Part model, mm, in its own coordinate system. A direction names the side the tool comes from. Coordinates: 2 decimals unless noted, no trailing zeros. Write each loop counter-clockwise with the first axis right and the second up, starting at its lowest first coordinate (ties: lowest second). Pieces come first, ordered by that corner, then holes. Notation, with made-up numbers: (-13.5, 80.25) - (8.5, 80.25) arc R24 ccw to (8.5, 111.25) - close; hole circle Ø2 at (86.25, 59.25). An arc over 180 degrees is marked (long way). Use a Markdown table: item, result.
```python
from build123d import *

# Parameters (mm, degrees)
SKETCH5_W            = 30
SKETCH5_H            = 80
BOSS_EXTRUDE4_DEPTH  = 20
SKETCH6_W            = 8
SKETCH6_H            = 5
BOSS_EXTRUDE5_DEPTH  = 5
SKETCH9_W            = 15
SKETCH9_H            = 22
BOSS_EXTRUDE10_DEPTH = 70
SKETCH14_W           = 15
SKETCH14_H           = 24
CUT_EXTRUDE1_DEPTH   = 18
FILLET1_R            = 2
FILLET2_R            = 10
FILLET4_R            = 2
FILLET6_R            = 2
SKETCH18_W           = 10
SKETCH18_H           = 18
BOSS_EXTRUDE11_DEPTH = 80
BOSS_EXTRUDE12_DEPTH = 10
CUT_EXTRUDE4_DEPTH   = 22


with BuildPart() as part:
    # Sketch5 → Boss-Extrude4 (new body)
    with BuildSketch(Plane(origin=(0, 0, 0), x_dir=(1, 0, 0), z_dir=(0, 1, 0))):
        Rectangle(SKETCH5_W, SKETCH5_H)
    extrude(amount=BOSS_EXTRUDE4_DEPTH)

    # Sketch6 → Boss-Extrude5 (add)
    with BuildSketch(Plane(origin=(0, 20, 0), x_dir=(1, 0, 0), z_dir=(0, 1, 0))):
        with Locations((8, 35.5)):
            Rectangle(SKETCH6_W, SKETCH6_H)
    extrude(amount=BOSS_EXTRUDE5_DEPTH)

    # Sketch9 → Boss-Extrude10 (add)
    with BuildSketch(Plane(origin=(0, 0, 0), x_dir=(1, 0, 0), z_dir=(0, 1, 0))):
        with Locations((-22.5, -24)):
            Rectangle(SKETCH9_W, SKETCH9_H)
    extrude(amount=BOSS_EXTRUDE10_DEPTH)

    # Sketch14 → Cut-Extrude1 (cut)
    with BuildSketch(Plane(origin=(0, 0, 13), x_dir=(-1, 0, 0), z_dir=(0, 0, -1))):
        with Locations((22.5, 54)):
            Rectangle(SKETCH14_W, SKETCH14_H)
    extrude(amount=-CUT_EXTRUDE1_DEPTH, mode=Mode.SUBTRACT)

    # Fillet1
    fillet1_edges = [part.edges().sort_by_distance(p)[0] for p in [
        (-15, 10, -40),
        (15, 10, -40),
        (15, 10, 40),
        (-15, 10, 40),
    ]]
    fillet(fillet1_edges, radius=FILLET1_R)

    # Fillet2
    fillet2_edges = [part.edges().sort_by_distance(p)[0] for p in [
        (-15, 10, 13),
    ]]
    fillet(fillet2_edges, radius=FILLET2_R)

    # Fillet4
    fillet4_edges = [part.edges().sort_by_distance(p)[0] for p in [
        (-30, 68, 13),
    ]]
    fillet(fillet4_edges, radius=FILLET4_R)

    # Fillet6
    fillet6_edges = [part.edges().sort_by_distance(p)[0] for p in [
        (-22.5, 70, 35),
        (-30, 70, 25),
        (-15, 70, 24),
        (-21.5, 70, 13),
        (-29.414213562, 70, 13.585786438),
    ]]
    fillet(fillet6_edges, radius=FILLET6_R)

    # Sketch18 → Boss-Extrude11 (add)
    with BuildSketch(Plane(origin=(0, 0, 0), x_dir=(-1, 0, 0), z_dir=(0, -1, 0))):
        with Locations((20, 13)):
            Rectangle(SKETCH18_W, SKETCH18_H)
    extrude(amount=-BOSS_EXTRUDE11_DEPTH)

    # Sketch19 → Boss-Extrude12 (add)
    with BuildSketch(Plane(origin=(0, 80, 0), x_dir=(1, 0, 0), z_dir=(0, 1, 0))):
        Polygon((-15, 22), (5, 22), (5, 14.741263634), (5, 6.741263634), (5, 4), (-15, 4), (-15, 6.741263634), (-15, 14.741263634), align=None)
    extrude(amount=-BOSS_EXTRUDE12_DEPTH)

    # Sketch20 → Cut-Extrude4 (cut)
    with BuildSketch(Plane(origin=(5, 0, 0), x_dir=(0, 0, -1), z_dir=(1, 0, 0))):
        Polygon((20, 80), (6, 80), (6, 78), (4, 78), (4, 72), (6, 72), (6, 70), (20, 70), (20, 72), (22, 72), (22, 78), (20, 78), align=None)
    extrude(amount=-CUT_EXTRUDE4_DEPTH, mode=Mode.SUBTRACT)


solid = part.part
```
Item 1: Two-plate mould, pull along Z, no slides. Class faces 5 (the face through (0, 10, 40)), 6 (the face through (-15, 10, 0)), 7 (the face through (4, 22, -35)): pulls with the +Z half, pulls with the -Z half, needs draft (parallel to the pull), parting line crosses it, or undercut.
From the geometry:
| item | result |
|---|---|
| face 5 | pulls with the +Z half |
| face 6 | undercut |
| face 7 | needs draft |
Item 2: Band-saw the part on D-D, the plane x = -21.5. Give the cut face in (y, z).
From the geometry:
| item | result |
|---|---|
| outline | (0, -22) - (80, -22) - (80, -4) - (0, -4) - close; (0, 12.37) - (20, 12.37) - (20, 13) - (42, 13) - (42, 31) - (66, 31) - (66, 13) - (68, 13) arc R2 ccw to (70, 15) - (70, 33) arc R2 ccw to (68, 35) - (0, 35) - close |
Item 3: Drop flat-ended pins along their axis: P1, Ø4, axis at x = 8, y = 21.5, coming from the -Z side; P2, Ø20, axis at y = 37.5, z = -9.5, coming from the +X side; P3, Ø1, axis at x = -16, z = -10, coming from the +Y side; P4, Ø12, axis at x = -22.5, y = 56, coming from the -Z side. Give the stop position or say it passes through.
From the geometry:
| item | result |
|---|---|
| P1 | z = -40 |
| P2 | x = -15 |
| P3 | y = 70 |
| P4 | z = -22 |
Item 4: Band-saw the part on C-C, the plane y = 65. Give the cut face in (x, z).
From the geometry:
| item | result |
|---|---|
| outline | (-30, 31) - (-15, 31) - (-15, 35) - (-30, 35) - close; (-25, -22) - (-15, -22) - (-15, -4) - (-25, -4) - close |
Item 5: Which spindle directions (+Z, -Z, +X, -X, +Y, -Y) get a long thin tool onto all of the face, cutting with end or side? Do faces 1 (the face through (-22, 67, 13)), 2 (the face through (-18.01, 10.14, 10.15)), 3 (the face through (-22, 66, 22)), 4 (the face through (-15, 33, 27)). Say none if no direction does.
From the geometry:
| item | result |
|---|---|
| face 1 | +X, -X, +Y |
| face 2 | -X, +Y, -Y |
| face 3 | +X, -X |
| face 4 | +Z, -Z, +X, +Y |
Item 6: Band-saw the part on B-B, the plane x = -1. Give the cut face in (y, z), then the cut area to 3 significant figures.
From the geometry:
| item | result |
|---|---|
| outline | (0, -40) - (20, -40) - (20, 40) - (0, 40) - close; (70, -22) - (72, -22) - (72, -20) - (70, -20) - close; (70, -6) - (72, -6) - (72, -4) - (70, -4) - close; (78, -22) - (80, -22) - (80, -20) - (78, -20) - close; (78, -6) - (80, -6) - (80, -4) - (78, -4) - close |
| area | 1,620 mm^2 |
Item 7: Drill centre lines: probe 1 along Z at (x, y) = (-10, 71.5); probe 2 along Z at (x, y) = (-22, 50); probe 3 along Y at (x, z) = (8, 19). Where is each one in solid material? Low to high.
From the geometry:
| item | result |
|---|---|
| probe 1 | -22 to -20, -6 to -4 |
| probe 2 | -22 to -4, 31 to 35 |
| probe 3 | 0 to 20 |
Item 8: Band-saw the part on A-A, the plane z = 25. Give the cut face in (x, y).
From the geometry:
| item | result |
|---|---|
| outline | (-30, 0) - (15, 0) - (15, 20) - (-15, 20) - (-15, 42) - (-30, 42) - close; (-30, 66) - (-15, 66) - (-15, 68) arc R2 ccw to (-17, 70) - (-28, 70) arc R2 ccw to (-30, 68) - close |
